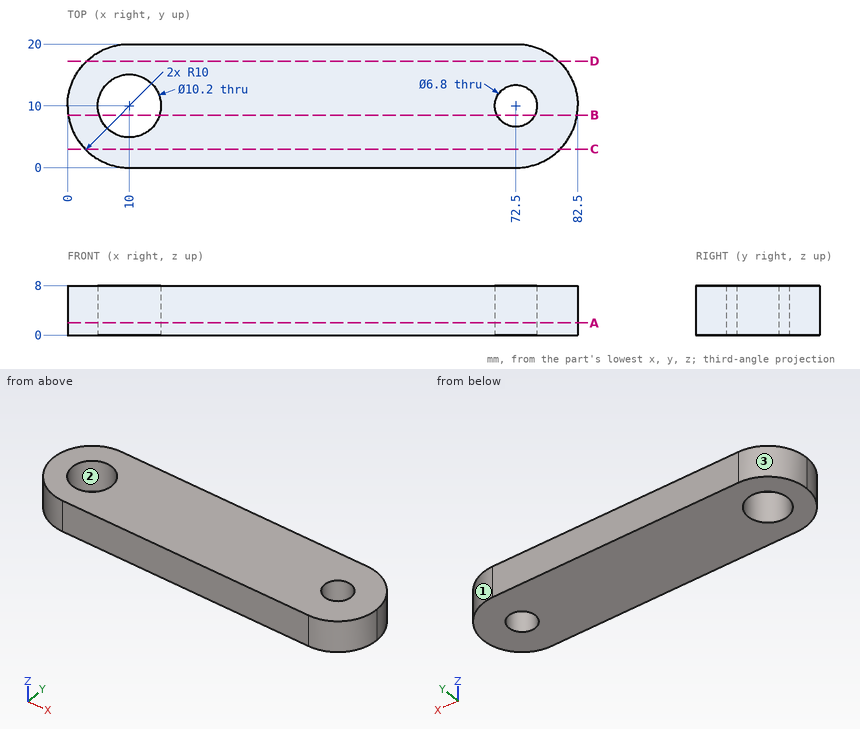
Geometry: see drawing. Coordinates: mm, zero at the bounding-box minimum. Round coordinates to 2 decimals unless told otherwise and drop trailing zeros. Loops run counter-clockwise (first coordinate to the right, second up) from the corner with the lowest first, then second, coordinate; pieces in that order, holes last. Notation, with made-up numbers: (42.25, -22.5) - (70.25, -22.5) arc R8 ccw to (70.25, -15.5) - close; hole circle Ø1 at (75, 22). An arc over 180 degrees is marked (long way). Write item = value, one per line. Start each with the question number.
(1) Section query A-A, the plane z = 2. State how many separate pieces and enclosed holes the cut face has, plus the area to 3 significant figures.
(2) Pull-direction query (X, two-part tool) for the marked faces 1, 2 and 3; classes: +X half, -X half, draft (parallel to the pull), parting line (faces both ways), or undercut.
(3) Ray query, line 1 along X through (y, z) = (9, 1); line 2 along Y through (x, z) = (10, 2.5); line 3 along Y through (x, z) = (7.5, 5.5). Return the intervals inside material, ascending. Write a range as from..to.
(4) Pin query (flat end, axial travel): pin 1 (1.5 mm diameter, centred on y = 5.5, z = 6, fed in from -X); pin 2 (3 mm diameter, centred on y = 4.5, z = 5, fed in from -X); pin 3 (1 mm diameter, centred on y = 4, z = 2.5, fed in from -X). Return the tip coordinate at first contact, or that it passes through.
(5) Section query D-D, the plane y = 17.25. Output: boundary loops of the cut face in (x, z).
(6) Section query C-C, the plane y = 3. Output: boundary loops of the cut face in (x, z).
(7) Section query B-B, the plane y = 8.5. Output: boundary loops of the cut face in (x, z), plus the area to 3 significant figures.
Conclusion:
q1.separate_pieces = 1
q1.enclosed_holes = 2
q1.area = 1,450 mm2
q2.face_1 = +X half
q2.face_2 = undercut
q2.face_3 = -X half
q3.line_1 = 0.05..5, 15..69.25, 75.75..82.45
q3.line_2 = 0..4.9, 15.1..20
q3.line_3 = 0.32..5.55, 14.45..19.68
q4.pin_1 = 0.73
q4.pin_2 = 0.83
q4.pin_3 = 1.65
q5.outline = (3.11, 0) - (79.39, 0) - (79.39, 8) - (3.11, 8) - close
q6.outline = (2.86, 0) - (79.64, 0) - (79.64, 8) - (2.86, 8) - close
q7.outline = (0.11, 0) - (5.13, 0) - (5.13, 8) - (0.11, 8) - close; (14.87, 0) - (69.45, 0) - (69.45, 8) - (14.87, 8) - close; (75.55, 0) - (82.39, 0) - (82.39, 8) - (75.55, 8) - close
q7.area = 531 mm2
